```python
from build123d import *

# Parameters (mm, degrees)
SKETCH1_R                = 2
BASE_FLANGE3_DEPTH       = 0.7366
SKETCHED_START           = -64
SKETCHED_BEND1_OUTLINE_W = 0.7366
SKETCHED_BEND1_OUTLINE_H = 65
SKETCHED_BEND1_DEPTH     = 64.108877104
SKETCHED_START_2         = 0.168203781
SKETCHED_BEND1_2_DEPTH   = 0.525916755
SKETCHED_START_3         = -0.042479464
SKETCHED_BEND1_3_DEPTH   = 1.4732
SKETCHED_START_4         = -32.5
SKETCHED_BEND1_4_DEPTH   = 65
SKETCH28_W               = 42.572846016
SKETCH28_H               = 16.402646855
CUT_EXTRUDE8_DEPTH       = 83.088587536
CUT_EXTRUDE9_DEPTH       = 83.088587536
CUT_EXTRUDE9_DEPTH_BACK  = 83.088587536
SKETCH29_R               = 1.725
SKETCH30_W               = 30
SKETCH30_H               = 65
SKETCH30_R               = 2
TAB1_DEPTH               = 0.7366


with BuildPart() as part:
    # Base-Flange3: sheet metal written as solids
    # Sketch1 → Base-Flange3 (new body)
    with BuildSketch(Plane(origin=(0, 0, 0), x_dir=(1, 0, 0), z_dir=(0, 1, 0))):
        with BuildLine():
            Line((-30.694120536, 32.5), (30.694120536, 32.5))
            Line((30.694120536, 32.5), (30.694120536, -32.5))
            Line((30.694120536, -32.5), (-30.694120536, -32.5))
            ThreePointArc((-30.694120536, -32.5), (-63.194120536, 0), (-30.694120536, 32.5))
        make_face()
        with Locations(Location((15.694120536, 0, 0), (0, 0, 270))):
            Circle(SKETCH1_R, mode=Mode.SUBTRACT)
    extrude(amount=-BASE_FLANGE3_DEPTH)

    # Sketched Bend1: read off the stored shape, not the designer's step
    # Sketched Bend1 outline → Sketched Bend1 (cut)
    with BuildSketch(Plane.YZ.offset(SKETCHED_START)):
        with Locations((-0.3683, 0)):
            Rectangle(SKETCHED_BEND1_OUTLINE_W, SKETCHED_BEND1_OUTLINE_H)
    extrude(amount=SKETCHED_BEND1_DEPTH, mode=Mode.SUBTRACT)

    # Sketched Bend1 2 outline → Sketched Bend1 2 (add)
    with BuildSketch(Plane.YZ.offset(SKETCHED_START_2)):
        with BuildLine():
            ThreePointArc((31.12586821, -32.5), (63.62586821, 0), (31.12586821, 32.5))
            Line((31.12586821, 32.5), (0, 32.5))
            Line((0, 32.5), (0, -32.5))
            Line((0, -32.5), (31.12586821, -32.5))
        make_face()
    extrude(amount=SKETCHED_BEND1_2_DEPTH)

    # Sketched Bend1 3 outline → Sketched Bend1 3 (add)
    with BuildSketch(Plane.YZ.offset(SKETCHED_START_3)):
        with BuildLine():
            ThreePointArc((31.12586821, -32.5), (63.62586821, 0), (31.12586821, 32.5))
            Line((31.12586821, 32.5), (0, 32.5))
            Line((0, 32.5), (0, -32.5))
            Line((0, -32.5), (31.12586821, -32.5))
        make_face()
    extrude(amount=SKETCHED_BEND1_3_DEPTH)

    # Sketched Bend1 4 outline → Sketched Bend1 4 (cut)
    with BuildSketch(Plane.XY.offset(SKETCHED_START_4)):
        with BuildLine():
            Line((0.694120536, 65), (0.694120536, 0.7366))
            ThreePointArc((0.694120536, 0.7366), (0.90986568, 0.215745144), (1.430720536, 0))
            Line((1.430720536, 0), (1.430720536, 65))
            Line((1.430720536, 65), (0.694120536, 65))
        make_face()
        with BuildLine():
            Line((-0.042479464, 0.7366), (-0.042479396, 65))
            Line((-0.042479396, 65), (-2, 65))
            Line((-2, 65), (-2, 0))
            Line((-2, 0), (0.108877104, 0))
            Line((0.108877104, 0), (0.108877104, -2))
            Line((0.108877104, -2), (32, -2))
            Line((32, -2), (32, -0.736599968))
            Line((32, -0.736599968), (1.430720536, -0.7366))
            ThreePointArc((1.430720536, -0.7366), (0.389010825, -0.30510971), (-0.042479464, 0.7366))
        make_face()
    extrude(amount=SKETCHED_BEND1_4_DEPTH, mode=Mode.SUBTRACT)

    # Sketch28 → Cut-Extrude8 (cut, through all)
    with BuildSketch(Plane.ZY.offset(9.729079464)):
        with Locations((5.381444798, 16.092801871)):
            Rectangle(SKETCH28_W, SKETCH28_H)
    extrude(amount=-CUT_EXTRUDE8_DEPTH, mode=Mode.SUBTRACT)

    # Sketch29 → Cut-Extrude9 (cut, two sides: drawn at the far end of the back side and taken through both)
    with BuildSketch(Plane.ZY.offset(9.729079464).offset(-CUT_EXTRUDE9_DEPTH_BACK)):
        with Locations(Location((-5.239369246, 44.083803898, 0), (0, 0, 270))):
            Circle(SKETCH29_R)
    extrude(amount=CUT_EXTRUDE9_DEPTH + CUT_EXTRUDE9_DEPTH_BACK, mode=Mode.SUBTRACT)

    # Tab1: sheet metal written as solids
    # Sketch30 → Tab1 (add)
    with BuildSketch(Plane(origin=(0, 0, 0), x_dir=(1, 0, 0), z_dir=(0, 1, 0))):
        with Locations((45.694120536, 0)):
            Rectangle(SKETCH30_W, SKETCH30_H)
        with Locations(Location((45.694120536, -17.5, 0), (0, 0, 270))):
            Circle(SKETCH30_R, mode=Mode.SUBTRACT)
        with Locations(Location((45.694120536, 17.5, 0), (0, 0, 270))):
            Circle(SKETCH30_R, mode=Mode.SUBTRACT)
    extrude(amount=-TAB1_DEPTH)


solid = part.part
```
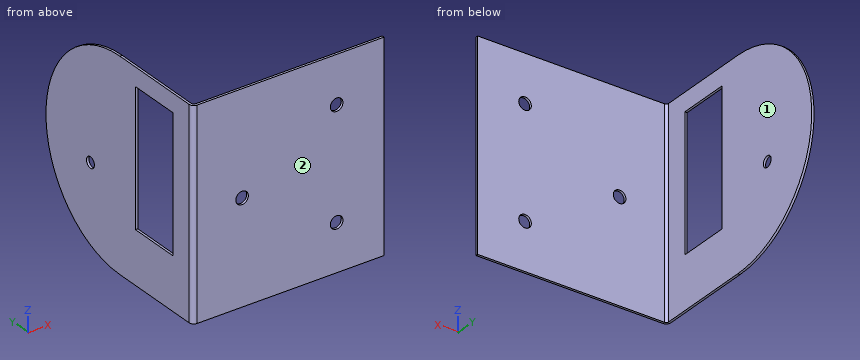
Could you check a few things on this model? Use its own coordinates, in mm. Face numbers are marked on the shaded views. A direction names the side the tool comes from. Round coordinates to 2 decimals unless told otherwise and drop trailing zeros. Loops run counter-clockwise (first coordinate to the right, second up) from the corner with the lowest first, then second, coordinate; pieces in that order, holes last. Notation, with made-up numbers: (-22, 1.25) - (6, 1.25) arc R29 cw to (6, 30.25) - close; hole circle Ø5 at (-6, 61.25). An arc over 180 degrees is marked (long way). Answer in a Markdown table with one row per item. Add a question column.
(1) For the marked faces 1 and 2, which set-ups out of +Z, -Z, +X, -X, +Y, -Y let a thin tool reach every point of the face, with its end or its side?
(2) If we section it at A-A (y = 23): Please give me the cut outline in (x, z), plus the area to 3 significant figures.
(3) If we section it at B-B (z = 0): Please give me the cut outline in (x, y), plus the area to 3 significant figures.
(4) If we section it at D-D (x = 52.5): Please give me the cut outline in (y, z).
(5) I'm going to push flat-ended pins straight in: pin 1 (6.5 mm diameter, centred on x = 15.69, z = 0, fed in from +Y); pin 2 (19 mm diameter, centred on y = 17.5, z = -15, fed in from +X); pin 3 (0.8 mm diameter, centred on x = 0.5, z = 9, fed in from -Y). Where does each tip first touch, or does it pass through?
(6) If we section it at C-C (z = 12): Please give me the cut outline in (x, y), plus the area to 3 significant figures.
(7) I need wall thicknesses on line 1 along Y through (x, z) = (24.5, -9); line 2 along X through (y, z) = (55.5, 2); line 3 along X through (y, z) = (-0.25, 0). Which ranges of each line are inside material? Lowest first, please.
Model answer:
| question | item | result |
|---|---|---|
| 1 | face 1 | +Z, -Z, +X, +Y |
| 1 | face 2 | +Z, -Z, +X, -X, -Y |
| 2 | outline | (-0.04, -32.5) - (0.69, -32.5) - (0.69, -15.9) - (-0.04, -15.9) - close; (-0.04, 26.67) - (0.69, 26.67) - (0.69, 32.5) - (-0.04, 32.5) - close |
| 2 | area | 16.5 mm² |
| 3 | outline | (-0.04, 0.74) arc R1.47 ccw to (1.43, -0.74) - (13.69, -0.74) - (13.69, 0) - (1.43, 0) arc R0.74 cw to (0.69, 0.74) - (0.69, 7.89) - (-0.04, 7.89) - close; (-0.04, 24.29) - (0.69, 24.29) - (0.69, 63.63) - (-0.04, 63.63) - close; (17.69, -0.74) - (60.69, -0.74) - (60.69, 0) - (17.69, 0) - close |
| 3 | area | 76.2 mm² |
| 4 | outline | (-0.74, -32.5) - (0, -32.5) - (0, 32.5) - (-0.74, 32.5) - close |
| 5 | pin 1 | stops at y = 0 |
| 5 | pin 2 | stops at x = 0.69 |
| 5 | pin 3 | stops at y = -0.64 |
| 6 | outline | (-0.04, 0.74) arc R1.47 ccw to (1.43, -0.74) - (60.69, -0.74) - (60.69, 0) - (1.43, 0) arc R0.74 cw to (0.69, 0.74) - (0.69, 7.89) - (-0.04, 7.89) - close; (-0.04, 24.29) - (0.69, 24.29) - (0.69, 61.33) - (-0.04, 61.33) - close |
| 6 | area | 77.5 mm² |
| 7 | line 1 | y = -0.74 to 0 |
| 7 | line 2 | x = -0.04 to 0.69 |
| 7 | line 3 | x = 0.34 to 13.69, 17.69 to 60.69 |
